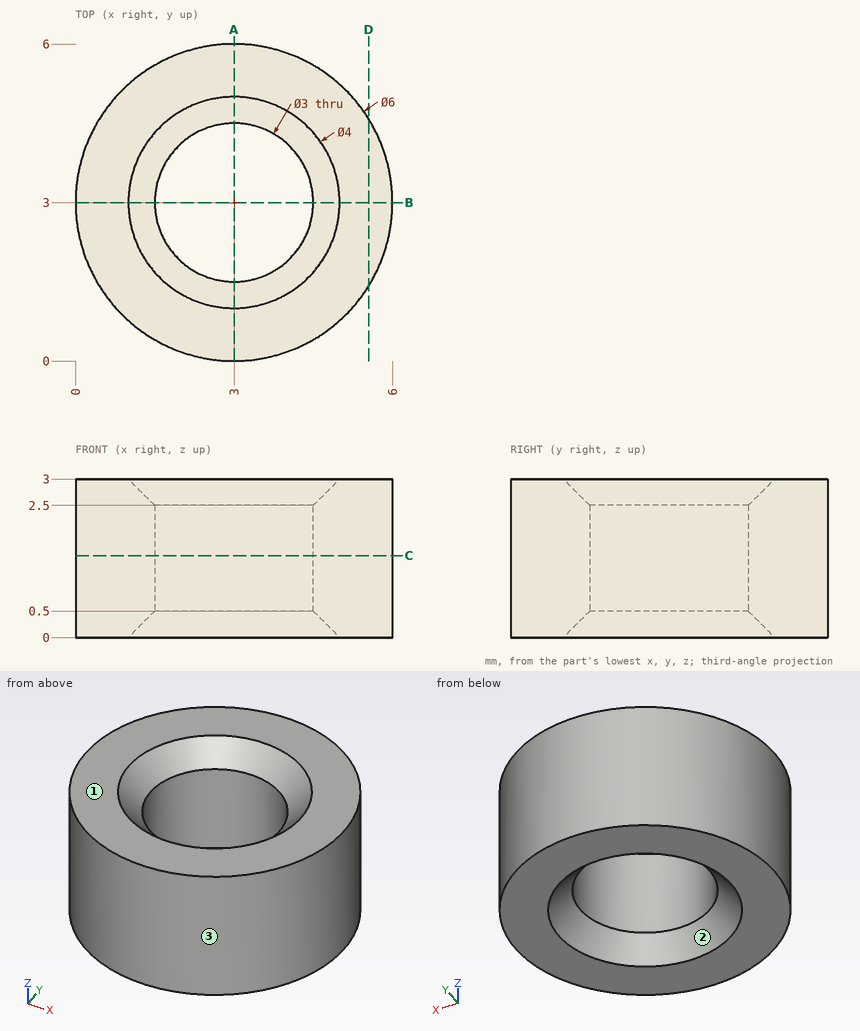
Geometry: see drawing. Coordinates: mm, zero at the bounding-box minimum. Give positions to 0.01 mm unless a question says otherwise; leave off trailing zeros. Order: outer loops, then holes, each group sorted by start corner. A loop starts at its lowest first (then second) coordinate and runs counter-clockwise, first axis right, second up. Notation, with made-up numbers: (-15, 36.5) -> (17, 36.5) arc R22 cw to (17, 68.5) -> close; hole circle Ø7 at (-33.75, 57). An arc over 180 degrees is marked (long way). Write item = value, one per line.
Q1. Cut plane D-D, the plane x = 5.55. Output: boundary loops of the cut face in (y, z), and give its area (3 significant figures).
Data:
outline = (1.42, 0) -> (4.58, 0) -> (4.58, 3) -> (1.42, 3) -> close
area = 9.48 mm^2
Q2. Cut plane C-C, the plane z = 1.55. Output: boundary loops of the cut face in (x, y).
Data:
outline = circle Ø6 at (3, 3); hole circle Ø3 at (3, 3)
Q3. Pull-direction query (X, two-part tool) for the marked faces 1, 2 and 3; classes: released by +X, released by -X, zero draft, split by the parting line, or undercut.
Data:
face_1 = zero draft
face_2 = undercut
face_3 = split by the parting line
Q4. Pin query (flat end, axial travel): pin 1 (1 mm diameter, centred on y = 5, z = 1, fed in from +X). Return the tip coordinate at first contact, or that it passes through.
Data:
pin_1 = 5.6
Q5. Material intervals for line 1 (Y direction, x = 3, z = 1.4); line 2 (X direction, y = 3.25, z = 1); line 3 (X direction, y = 2.7, z = 2.6), sorted ascending. Write a range as from..to.
Data:
line_1 = 0..1.5, 4.5..6
line_2 = 0.01..1.52, 4.48..5.99
line_3 = 0.02..1.43, 4.57..5.98
Q6. Cut plane A-A, the plane x = 3. Output: boundary loops of the cut face in (y, z).
Data:
outline = (0, 0) -> (1, 0) -> (1.5, 0.5) -> (1.5, 2.5) -> (1, 3) -> (0, 3) -> close; (4.5, 0.5) -> (5, 0) -> (6, 0) -> (6, 3) -> (5, 3) -> (4.5, 2.5) -> close
